Drawing for the job (mm, zero at the part's lowest x, y, z). Give positions to 0.01 mm unless a question says otherwise; leave off trailing zeros. Order: outer loops, then holes, each group sorted by start corner. A loop starts at its lowest first (then second) coordinate and runs counter-clockwise, first axis right, second up. Notation, with made-up numbers: M 35.25,44.5 L 86.25,44.5 A22 ccw 86.25,56.5 Z; hole C 35,24 d11. An arc over 180 degrees is marked long. Answer as a JSON object with one key per item and string values.
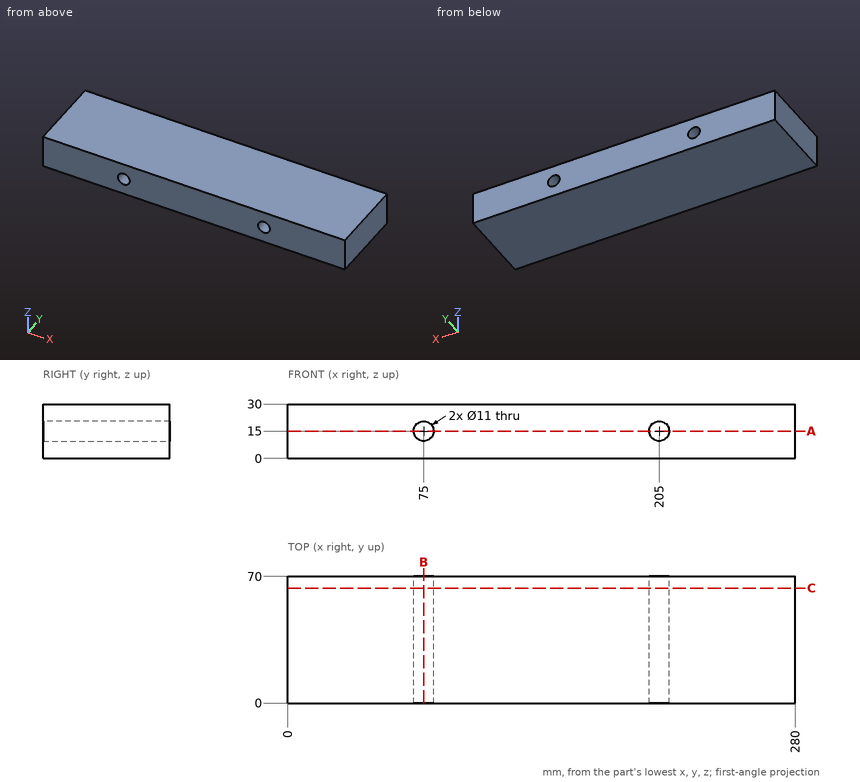
1. Cut at C-C on y = 63.5. Give the cut face in (x, z), plus the area to 3 significant figures.
Worked answers:
{"outline": "M 0,0 L 280,0 L 280,30 L 0,30 Z; hole C 75,15 d11; hole C 205,15 d11", "area": "8,210 mm^2"}
2. Cut at A-A on z = 15. Give the cut face in (x, y).
Worked answers:
{"outline": "M 0,0 L 69.5,0 L 69.5,70 L 0,70 Z; M 80.5,0 L 199.5,0 L 199.5,70 L 80.5,70 Z; M 210.5,0 L 280,0 L 280,70 L 210.5,70 Z"}
3. Cut at B-B on x = 75. Give the cut face in (y, z), plus the area to 3 significant figures.
Worked answers:
{"outline": "M 0,0 L 70,0 L 70,9.5 L 0,9.5 Z; M 0,20.5 L 70,20.5 L 70,30 L 0,30 Z", "area": "1,330 mm^2"}
4. Probe line 1 along X through (y, z) = (31, 15); line 2 along X through (y, z) = (20.5, 15.75); line 3 along Z through (x, y) = (207, 30). List the from-to ranges inside material, lowest first.
Worked answers:
{"line 1": "x = 0 to 69.5, 80.5 to 199.5, 210.5 to 280", "line 2": "x = 0 to 69.55, 80.45 to 199.55, 210.45 to 280", "line 3": "z = 0 to 9.88, 20.12 to 30"}
